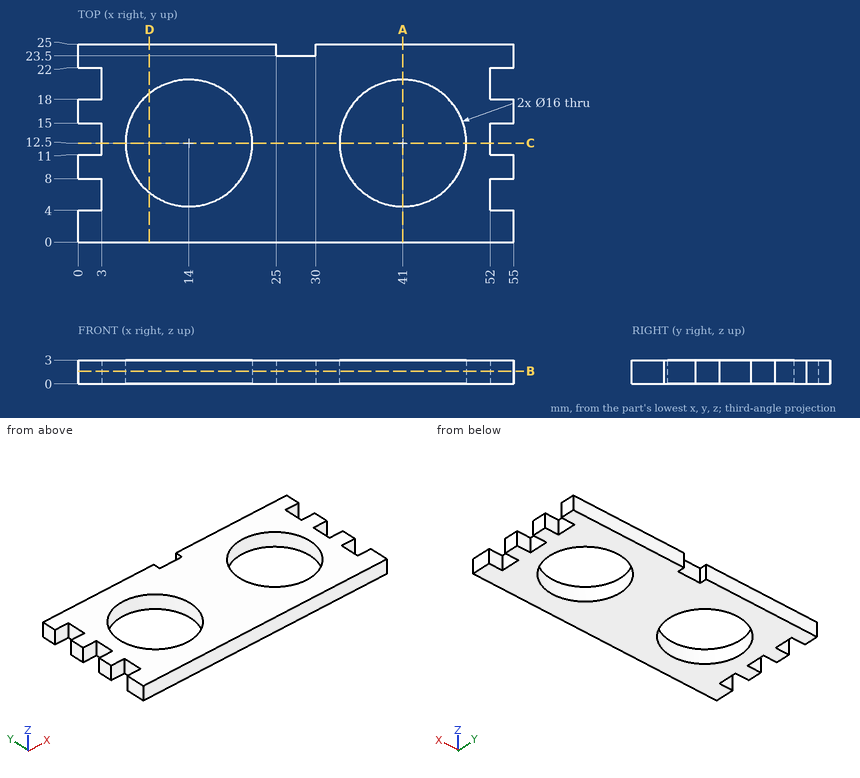
Here's the drawing with two shaded views (mm, measured from the low corner). I have some questions. Round coordinates to 2 decimals unless told otherwise and drop trailing zeros. Loops run counter-clockwise (first coordinate to the right, second up) from the corner with the lowest first, then second, coordinate; pieces in that order, holes last.
1. Suppose I cut it at D-D, the plane x = 9. Please give me the cut outline in (y, z) (3 decimals), and give its area (3 significant figures).
Answers:
outline: (0, 0) - (6.255, 0) - (6.255, 3) - (0, 3) - close; (18.745, 0) - (25, 0) - (25, 3) - (18.745, 3) - close
area: 37.5 mm2
2. Suppose I cut it at A-A, the plane x = 41. Please give me the cut outline in (y, z).
Answers:
outline: (0, 0) - (4.5, 0) - (4.5, 3) - (0, 3) - close; (20.5, 0) - (25, 0) - (25, 3) - (20.5, 3) - close
3. If I drill on probe 1 along X at (y, z) = (24, 2.8); probe 2 along Y at (x, z) = (41, 1.85); probe 3 along X at (y, z) = (7, 0.4), over which ranges is the centre line in solid material (lowest first)?
Answers:
probe 1: x = 0 to 25, 30 to 55
probe 2: y = 0 to 4.5, 20.5 to 25
probe 3: x = 3 to 8.19, 19.81 to 35.19, 46.81 to 52
4. Suppose I cut it at C-C, the plane y = 12.5. Please give me the cut outline in (x, z).
Answers:
outline: (3, 0) - (6, 0) - (6, 3) - (3, 3) - close; (22, 0) - (33, 0) - (33, 3) - (22, 3) - close; (49, 0) - (52, 0) - (52, 3) - (49, 3) - close
5. Suppose I cut it at B-B, the plane z = 1.6. Give the number of separate pieces and of enclosed holes in the cut face, and give its area (3 significant figures).
Answers:
separate pieces: 1
enclosed holes: 2
area: 893 mm2
6. Will these pins go through, and if not, where does the flat tip stop? pin 1 (13 mm diameter, centred on x = 41, y = 12.5, fed in from -Z); pin 2 (0.9 mm diameter, centred on y = 6.5, z = 1.5, fed in from -X); pin 3 (0.9 mm diameter, centred on y = 13.5, z = 1, fed in from +X).
Answers:
pin 1: passes through
pin 2: stops at x = 3
pin 3: stops at x = 52
